Drawing for the job (mm, zero at the part's lowest x, y, z). Round coordinates to 2 decimals unless told otherwise and drop trailing zeros. Write each loop counter-clockwise with the first axis right and the second up, starting at its lowest first coordinate (ties: lowest second). Pieces come first, ordered by that corner, then holes. Notation, with made-up numbers: (38.25, 54.25) - (70.25, 54.25) arc R17 ccw to (70.25, 71.25) - close; hole circle Ø4 at (23, 66). An arc over 180 degrees is marked (long way). One line per question, with ' | ' between items.
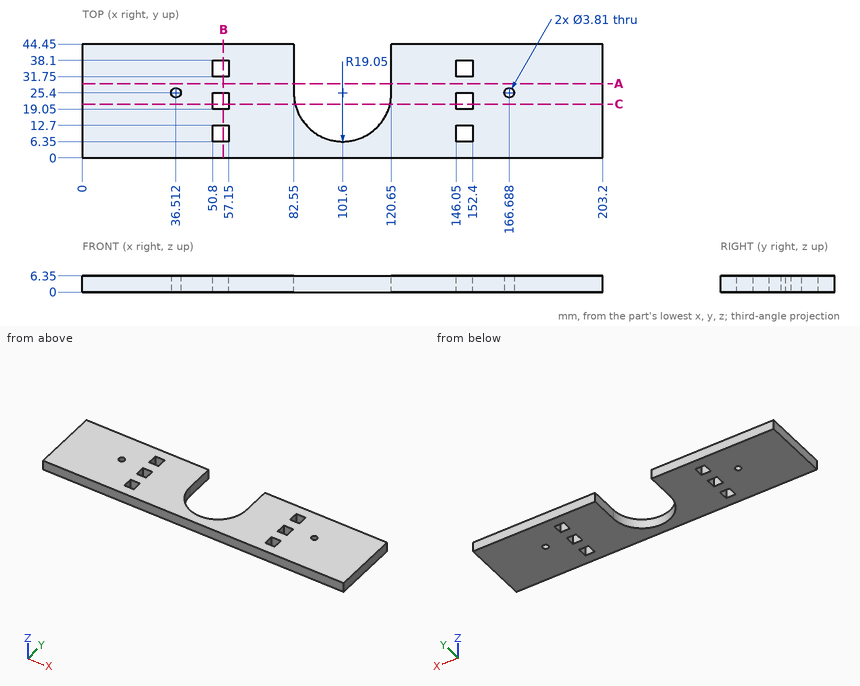
Q1. Saw through at B-B, the plane x = 55. List the corners of the cut face in (y, z), then the cut area to 3 significant figures.
Found:
outline: (0, 0) - (6.35, 0) - (6.35, 6.35) - (0, 6.35) - close; (12.7, 0) - (19.05, 0) - (19.05, 6.35) - (12.7, 6.35) - close; (25.4, 0) - (31.75, 0) - (31.75, 6.35) - (25.4, 6.35) - close; (38.1, 0) - (44.45, 0) - (44.45, 6.35) - (38.1, 6.35) - close | area: 161 mm^2
Q2. Saw through at C-C, the plane y = 21. State how many separate pieces and enclosed holes the cut face has.
Found:
separate pieces: 4 | enclosed holes: 0
Q3. Drill centre lines: L1, parallel to X at y = 28, z = 2; L2, parallel to X at y = 33.5, z = 0.5; L3, parallel to X at y = 19.5, z = 2. Where is each one in solid material? Low to high. Write a range as from..to.
Found:
L1: 0..82.55, 120.65..203.2 | L2: 0..50.8, 57.15..82.55, 120.65..146.05, 152.4..203.2 | L3: 0..50.8, 57.15..83.49, 119.71..146.05, 152.4..203.2
Q4. Saw through at A-A, the plane y = 29. List the corners of the cut face in (x, z), then the cut area to 3 significant figures.
Found:
outline: (0, 0) - (82.55, 0) - (82.55, 6.35) - (0, 6.35) - close; (120.65, 0) - (203.2, 0) - (203.2, 6.35) - (120.65, 6.35) - close | area: 1,050 mm^2
